The model under review builds one solid part; all positions refer to its coordinate system, in mm. A direction names the side the tool comes from. Round coordinates to 2 decimals unless told otherwise and drop trailing zeros. Loops run counter-clockwise (first coordinate to the right, second up) from the corner with the lowest first, then second, coordinate; pieces in that order, holes last. Notation, with made-up numbers: (-18.75, 2.5) -> (27.25, 2.5) arc R34 ccw to (27.25, 36.5) -> close; hole circle Ø10 at (9, -38.75). An arc over 180 degrees is marked (long way). Use a Markdown table: item, result. Add a question column.
1) Insertion check: pin 1 (3 mm diameter, centred on y = -27.5, z = 43.5, fed in from +X); pin 2 (1.5 mm diameter, centred on x = 43.5, y = -13, fed in from +Z); pin 3 (10 mm diameter, centred on y = -14, z = 38, fed in from -X). Each pin has a flat end and moves straight along its axis. Give the tip position at first contact, or say it passes through.
2) Consider section A-A on x = 24. Give the boundary of the cut face in (y, z), plus the area to 3 significant figures.
3) For faces 1 (the flat face through (31, -21.589, 2)), 2 (the cylindrical face through (-32.746, -7.333, 36.715)), list the 3-axis set-ups (+Z, -Z, +X, -X, +Y, -Y) from which the entire face can be reached by the end or side of a thin tool; tool diameter is ignored.
4) Wall thickness on probe 1 along Z at (x, y) = (-28.5, -36); probe 2 along Z at (x, y) = (34.5, -26); probe 3 along Z at (x, y) = (-36.5, -27): over which ranges is each line inside the solid? List them lowest first.
5) Mouldability with a two-part tool opening along Z and no side actions: class faces 3 (the cylindrical face through (63.2, -18.8, 2.3)), 4 (the flat face through (-31.416, -18.783, 34.609)), 5 (the flat face through (-3, -38.1, 3)), 6 (the cylindrical face through (-32.75, -25.53, 36.71)) as released by +Z, released by -Z, zero draft, split by the parting line, or undercut.
6) Consider section B-B on y = -11. Give the boundary of the cut face in (x, z).
7) Consider section D-D on x = -24.5. Give the boundary of the cut face in (y, z).
8) Consider section C-C on y = -36. Give the boundary of the cut face in (x, z), plus the area to 3 significant figures.
from build123d import *

# Parameters (mm, degrees)
F1_DEPTH = 38.1
F2_R     = 5.5756630796
F3_DEPTH = 25.4
F4_R     = 3.175
F5_DEPTH = 25.4


with BuildPart() as f1:
    # F0 (on Front) → F1 (new body)
    with BuildSketch(Plane.XZ):
        with BuildLine():
            Line((-32.8956767917, 0), (60.8509816229, 0))
            ThreePointArc((60.8509816229, 0), (63.2006728556, 2.3496912327), (60.8509816229, 4.6993824653))
            Line((60.8509816229, 4.6993824653), (-32.8956767917, 4.6993824653))
            ThreePointArc((-32.8956767917, 4.6993824653), (-39.2909683128, 8.4415319313), (-39.1615219414, 15.8500864396))
            Line((-39.1615219414, 15.8500864396), (-23.4511158537, 53.9007586853))
            ThreePointArc((-23.4511158537, 53.9007586853), (-24.5476949895, 56.5224848042), (-27.1643130178, 55.4137721553))
            Line((-27.1643130178, 55.4137721553), (-43.4994138777, 15.8500864396))
            ThreePointArc((-43.4994138777, 15.8500864396), (-42.43067129, 5.0930741417), (-32.8956767917, 0))
        make_face()
    extrude(amount=F1_DEPTH)

    # F2 (on face) → F3 (cut)
    with BuildSketch(Plane.XY.offset(4.6993824653)):
        with Locations((-10.7061062008, -18.751559779)):
            Circle(F2_R)
        with BuildLine():
            Line((46.6441214085, -15.3064941987), (16.8544258922, -15.3064941987))
            ThreePointArc((16.8544258922, -15.3064941987), (13.5090501422, -18.3429366679), (16.6517738253, -21.5886738151))
            Line((16.6517738253, -21.5886738151), (46.6441214085, -21.5886738151))
            ThreePointArc((46.6441214085, -21.5886738151), (49.7852112167, -18.4475840069), (46.6441214085, -15.3064941987))
        make_face()
    extrude(amount=-F3_DEPTH, mode=Mode.SUBTRACT)

    # F4 (on face) → F5 (cut)
    with BuildSketch(Plane(origin=(-42.7551148795, 0, 17.6527818681), x_dir=(0, -1, 0), z_dir=(-0.9243143528, 0, 0.3816319917))):
        with Locations((9.8523907273, 23.3707670122)):
            Circle(F4_R)
        with Locations((28.044729707, 23.3707670122)):
            Circle(F4_R)
    extrude(amount=-F5_DEPTH, mode=Mode.SUBTRACT)


solid = f1.part
Result set:
| question | item | result |
|---|---|---|
| 1 | pin 1 | x = -27.13 |
| 1 | pin 2 | z = 4.7 |
| 1 | pin 3 | x = -36.42 |
| 2 | outline | (-38.1, 0) -> (-21.59, 0) -> (-21.59, 4.7) -> (-38.1, 4.7) -> close; (-15.31, 0) -> (0, 0) -> (0, 4.7) -> (-15.31, 4.7) -> close |
| 2 | area | 150 mm2 |
| 3 | face 1 | +Z, -Z |
| 3 | face 2 | none |
| 4 | probe 1 | 0 to 4.7, 41.67 to 52.18 |
| 4 | probe 2 | 0 to 4.7 |
| 4 | probe 3 | 0.58 to 5.65, 22.3 to 32.8 |
| 5 | face 3 | split by the parting line |
| 5 | face 4 | undercut |
| 5 | face 5 | zero draft |
| 5 | face 6 | undercut |
| 6 | outline | (-43.5, 15.85) arc R11.47 ccw to (-32.9, 0) -> (60.85, 0) arc R2.35 ccw to (60.85, 4.7) -> (-32.9, 4.7) arc R7.34 cw to (-39.16, 15.85) -> (-31.26, 34.99) -> (-34.97, 36.52) -> close; (-32.71, 41.99) -> (-29, 40.46) -> (-23.45, 53.9) arc R2 ccw (long way) to (-27.16, 55.41) -> close |
| 7 | outline | (-38.1, 0) -> (0, 0) -> (0, 4.7) -> (-38.1, 4.7) -> close; (-38.1, 51.36) -> (0, 51.36) -> (0, 56.5) -> (-38.1, 56.5) -> close |
| 8 | outline | (-43.5, 15.85) arc R11.47 ccw to (-32.9, 0) -> (60.85, 0) arc R2.35 ccw to (60.85, 4.7) -> (-32.9, 4.7) arc R7.34 cw to (-39.16, 15.85) -> (-23.45, 53.9) arc R2 ccw (long way) to (-27.16, 55.41) -> close |
| 8 | area | 707 mm2 |
